Geometry check sheet. Reference: drawing and pictorial views, mm from the part's lowest x, y, z. A direction names the side the tool comes from. Coordinates: 2 decimals unless noted, no trailing zeros. Loops run counter-clockwise (first coordinate to the right, second up) from the corner with the lowest first, then second, coordinate; pieces in that order, holes last.
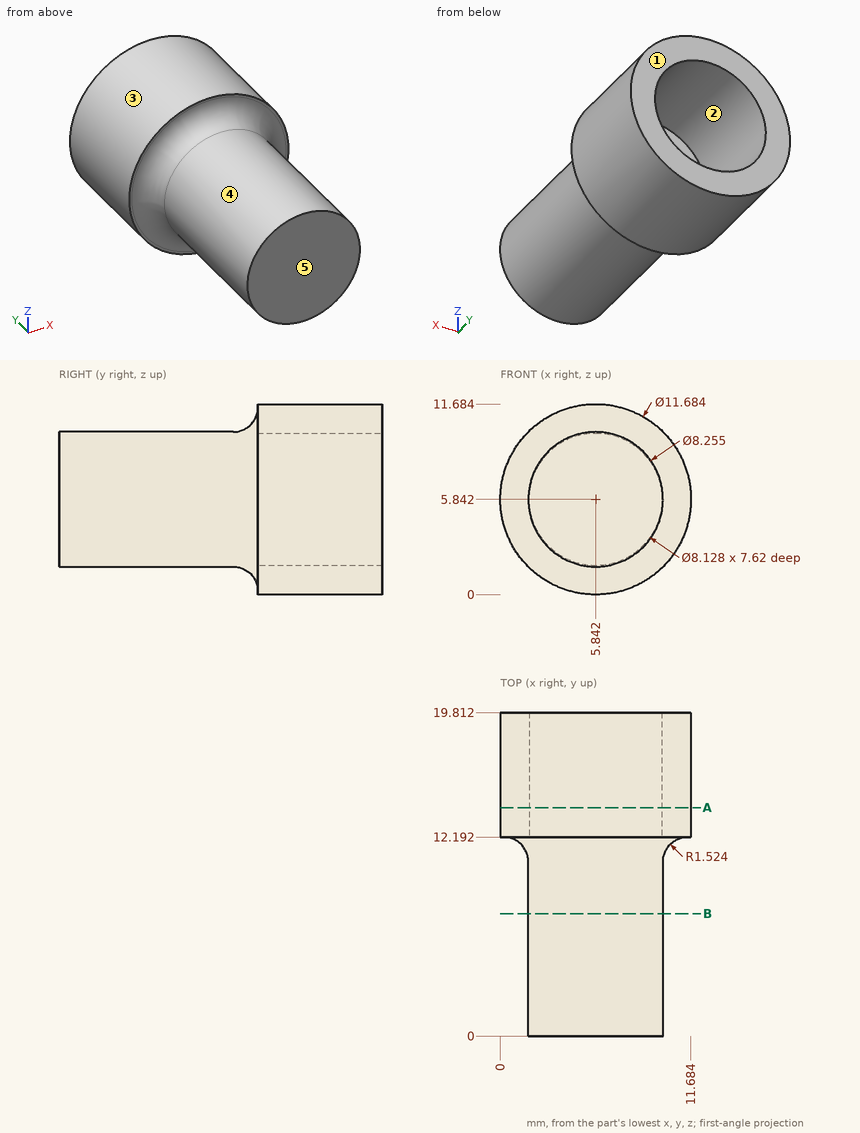
1) Section check A-A on y = 14. Record the cut outline in (x, z), and give its area (3 significant figures).
Data:
outline: circle Ø11.68 at (5.84, 5.84); hole circle Ø8.13 at (5.84, 5.84)
area: 55.3 mm2
2) Depth check by flat-ended pin: pin 1 (5 mm diameter, centred on y = 13, z = 10, fed in from +X); pin 2 (3 mm diameter, centred on y = 5, z = 2, fed in from -X); pin 3 (1.5 mm diameter, centred on y = 2.5, z = 6, fed in from +X); pin 4 (3.5 mm diameter, centred on x = 7, z = 4, fed in from -Y). Enter the tip coordinate at first touch or a pass-through.
Data:
pin 1: stops at x = 11.44
pin 2: stops at x = 2.44
pin 3: stops at x = 9.97
pin 4: stops at y = 0
3) Material ranges on probe 1 along Y at (x, z) = (4.5, 10); probe 2 along Y at (x, z) = (7.25, 3); probe 3 along X at (y, z) = (18.25, 7.75), recorded low to high.
Data:
probe 1: y = 11.49 to 19.81
probe 2: y = 0 to 12.19
probe 3: x = 0.32 to 2.25, 9.43 to 11.36
4) Mould release check, pull along Z, two halves, no side actions. Record for the marked faces 1, 2 and 3: +Z half, -Z half, draft (parallel to the pull), parting line (faces both ways), or undercut.
Data:
face 1: draft
face 2: undercut
face 3: parting line
5) Access from +Z, -Z, +X, -X, +Y, -Y to the whole of each face (thin tool, end or side, straight path). Record for the marked faces 4 and 5.
Data:
face 4: -Y
face 5: +Z, -Z, +X, -X, -Y
6) Section check B-B on y = 7.5. Record the cut outline in (x, z) (1 decimal).
Data:
outline: circle Ø8.3 at (5.8, 5.8)
